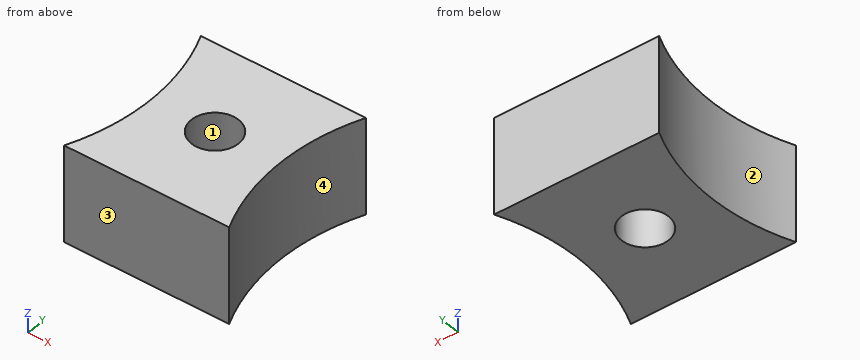
from build123d import *

# Parameters (mm, degrees)
F0_R     = 10
F1_DEPTH = 41.1


# Not quite as in the source:
# - a feature names something its author has since deleted; it is built from what else it names


with BuildPart() as f1:
    # F0 (on Top) → F1 (new body)
    with BuildSketch(Plane.XY):
        with BuildLine():
            ThreePointArc((-34.6869575489, 36.5), (-27, 0), (-34.6869575489, -36.5))
            Line((-34.6869575489, -36.5), (34.6869575489, -36.5))
            ThreePointArc((34.6869575489, -36.5), (27, 0), (34.6869575489, 36.5))
            Line((34.6869575489, 36.5), (-34.6869575489, 36.5))
        make_face()
        Circle(F0_R, mode=Mode.SUBTRACT)
    extrude(amount=F1_DEPTH)


solid = f1.part
Geometry: final body of the model. Coordinates: model frame, mm. Face numbers are marked on the shaded views. Give positions to 0.01 mm unless a question says otherwise; leave off trailing zeros. Write each loop counter-clockwise with the first axis right and the second up, starting at its lowest first coordinate (ties: lowest second). Pieces come first, ordered by that corner, then holes. Notation, with made-up numbers: M 34.25,56.5 L 78.25,56.5 A22 cw 78.25,93.5 Z; hole C -38.5,-1.75 d10. An arc over 180 degrees is marked long. Answer in a Markdown table with one row per item. Add a question column.
(1) Mould query, pull axis X, two halves, no side actions, for the marked faces 1, 2, 3 and 4. Classes: +X half, -X half, draft (parallel to the pull), parting line (faces both ways), or undercut.
(2) Section A-A on x = 0. Return loops of the section in (y, z), and give its area (3 significant figures).
(3) First-contact query: pin 1 (12 mm diameter, centred on y = -16.5, z = 20, fed in from +X); pin 2 (3 mm diameter, centred on y = -10, z = 23, fed in from -X); pin 3 (8 mm diameter, centred on y = 28, z = 33, fed in from -X); pin 4 (12 mm diameter, centred on x = 0, y = 0, fed in from +Z). Flat tips, straight axial feed; report the tip coordinate or a pass-through.
(4) Section D-D on y = 22.5. Return loops of the section in (x, z).
(5) Section B-B on y = 0. Return loops of the section in (x, z).
(6) Section C-C on z = 25. Return loops of the section in (x, y), and give its area (3 significant figures).
(7) Ray query, line 1 (Y direction, x = 0, z = 25.5); line 2 (X direction, y = 0.5, z = 13); line 3 (Y direction, x = 2, z = 12.5). Return the intervals inside material, ascending.
Result set:
| question | item | result |
|---|---|---|
| 1 | face 1 | undercut |
| 1 | face 2 | -X half |
| 1 | face 3 | draft |
| 1 | face 4 | +X half |
| 2 | outline | M -36.5,0 L -10,0 L -10,41.1 L -36.5,41.1 Z; M 10,0 L 36.5,0 L 36.5,41.1 L 10,41.1 Z |
| 2 | area | 2,180 mm^2 |
| 3 | pin 1 | stops at x = 29.84 |
| 3 | pin 2 | stops at x = -27.73 |
| 3 | pin 3 | stops at x = -32.85 |
| 3 | pin 4 | passes through |
| 4 | outline | M -29.84,0 L 29.84,0 L 29.84,41.1 L -29.84,41.1 Z |
| 5 | outline | M -27,0 L -10,0 L -10,41.1 L -27,41.1 Z; M 10,0 L 27,0 L 27,41.1 L 10,41.1 Z |
| 6 | outline | M -34.69,-36.5 L 34.69,-36.5 A90.5 cw 34.69,36.5 L -34.69,36.5 A90.5 cw Z; hole C 0,0 d20 |
| 6 | area | 4,000 mm^2 |
| 7 | line 1 | y = -36.5 to -10, 10 to 36.5 |
| 7 | line 2 | x = -27 to -9.99, 9.99 to 27 |
| 7 | line 3 | y = -36.5 to -9.8, 9.8 to 36.5 |
